Could you check a few things on this model? Use its own coordinates, in mm. Round coordinates to 2 decimals unless told otherwise and drop trailing zeros. Write each loop counter-clockwise with the first axis right and the second up, starting at its lowest first coordinate (ties: lowest second). Pieces come first, ordered by that corner, then holes.
```python
from build123d import *

# Parameters (mm, degrees)
EXTRUDE_START        = 90
SKETCH_1_R           = 1.65
EXTRUDE_262_DEPTH    = 2
EXTRUDE_START_2      = 4
EXTRUDE_1_DEPTH      = 4
D3P2_1_START         = 2
SKETCH_3_R           = 1.6
D3P2_1_DEPTH         = 2
EXTRUDE_1_2_DEPTH    = 4
SKETCH_5_R           = 1.6
D3P2_1_2_DEPTH       = 2
CUT_EXTRUDE_START    = 90
CUT_EXTRUDE_45_DEPTH = 2


with BuildPart() as part:
    # 草图1 → Extrude 262 (new body)
    with BuildSketch(Plane(origin=(0, 0, 0), x_dir=(1, 0, 0), z_dir=(0, 1, 0)).offset(EXTRUDE_START)):
        Polygon((-22.5, -3.5), (-22.5, -12), (-24.25, -15), (-24.25, -53), (-21.25, -56), (-5, -56), (-5, -59), (5, -59), (5, -56), (21.25, -56), (24.25, -53), (24.25, -15), (22.5, -12), (22.5, -3.5), align=None)
        with Locations(Location((0, -56.5, 0), (0, 0, 270))):
            Circle(SKETCH_1_R, mode=Mode.SUBTRACT)
    extrude(amount=EXTRUDE_262_DEPTH)

    # 草图2 → Extrude 1 (add)
    with BuildSketch(Plane.XY.offset(EXTRUDE_START_2)):
        with BuildLine():
            Line((-20.5, 88), (-15.5, 88))
            ThreePointArc((-15.5, 88), (-15.146446609, 88.146446609), (-15, 88.5))
            Line((-15, 88.5), (-15, 89.5))
            ThreePointArc((-15, 89.5), (-15.146446609, 89.853553391), (-15.5, 90))
            Line((-15.5, 90), (-20.5, 90))
            ThreePointArc((-20.5, 90), (-20.853553391, 89.853553391), (-21, 89.5))
            Line((-21, 89.5), (-21, 88.5))
            ThreePointArc((-21, 88.5), (-20.853553391, 88.146446609), (-20.5, 88))
        make_face()
    extrude(amount=EXTRUDE_1_DEPTH)

    # 草图3 → D3p2_-1 (add)
    with BuildSketch(Plane.XY.offset(D3P2_1_START)):
        with Locations(Location((-18, 89, 0), (0, 0, 218.682187453))):
            Circle(SKETCH_3_R)
    extrude(amount=D3P2_1_DEPTH)

    # 草图4 → Extrude 1 2 (add)
    with BuildSketch(Plane.XY.offset(EXTRUDE_START_2)):
        with BuildLine():
            Line((15.5, 88), (20.5, 88))
            ThreePointArc((20.5, 88), (20.853553391, 88.146446609), (21, 88.5))
            Line((21, 88.5), (21, 89.5))
            ThreePointArc((21, 89.5), (20.853553391, 89.853553391), (20.5, 90))
            Line((20.5, 90), (15.5, 90))
            ThreePointArc((15.5, 90), (15.146446609, 89.853553391), (15, 89.5))
            Line((15, 89.5), (15, 88.5))
            ThreePointArc((15, 88.5), (15.146446609, 88.146446609), (15.5, 88))
        make_face()
    extrude(amount=EXTRUDE_1_2_DEPTH)

    # 草图5 → D3p2_1 2 (add)
    with BuildSketch(Plane.XY.offset(D3P2_1_START)):
        with Locations(Location((18, 89, 0), (0, 0, 218.682187453))):
            Circle(SKETCH_5_R)
    extrude(amount=D3P2_1_2_DEPTH)

    # 草图6 → 后盖45度平行通气孔 (cut)
    with BuildSketch(Plane(origin=(0, 0, 0), x_dir=(1, 0, 0), z_dir=(0, 1, 0)).offset(CUT_EXTRUDE_START)):
        with BuildLine():
            Line((-1.767766953, -21.464466094), (3.535533906, -26.767766953))
            ThreePointArc((3.535533906, -26.767766953), (3.535533906, -28.535533906), (1.767766953, -28.535533906))
            Line((1.767766953, -28.535533906), (-3.535533906, -23.232233047))
            ThreePointArc((-3.535533906, -23.232233047), (-3.535533906, -21.464466094), (-1.767766953, -21.464466094))
        make_face()
        with BuildLine():
            Line((-1.767766953, -27.464466094), (3.535533906, -32.767766953))
            ThreePointArc((3.535533906, -32.767766953), (3.535533906, -34.535533906), (1.767766953, -34.535533906))
            Line((1.767766953, -34.535533906), (-3.535533906, -29.232233047))
            ThreePointArc((-3.535533906, -29.232233047), (-3.535533906, -27.464466094), (-1.767766953, -27.464466094))
        make_face()
    extrude(amount=CUT_EXTRUDE_45_DEPTH, mode=Mode.SUBTRACT)


solid = part.part
```
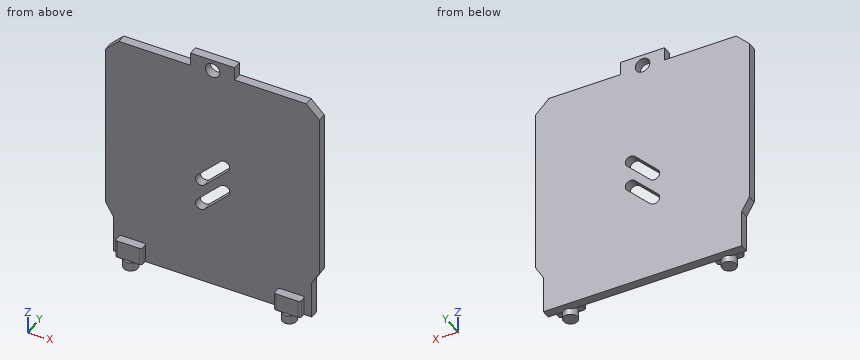
Q1. Imagine slicing it at D-D, the plane z = 19. Write out the boundary of the cut face in (x, y).
Q2. Imagine slicing it at A-A, the plane x = 0. Write out the boundary of the cut face in (y, z).
Q3. I'm going to push flat-ended pins straight in: pin 1 Ø0.6 at (x, y) = (13.5, 90.5) entering from +Z; pin 2 Ø1.6 at (y, z) = (90.5, 57) entering from +X; pin 3 Ø2 at (y, z) = (91, 9) entering from +X. Where does each tip first touch, or does it pass through?
Q4. Imagine slicing it at C-C, the plane x = -18. Write out the boundary of the cut face in (y, z), then the cut area to 3 significant figures.
Q5. Imagine slicing it at B-B, the plane z = 25. Write out the boundary of the cut face in (x, y), then the cut area to 3 significant figures.
Q6. If I drill on L1, parallel to X at y = 91.15, z = 56.5; L2, parallel to X at y = 88.95, z = 6; L3, parallel to Y at x = -4, z = 51, over which ranges is the centre line in solid material (lowest first)?
Results found:
1. outline: (-24.25, 90) - (24.25, 90) - (24.25, 92) - (-24.25, 92) - close
2. outline: (90, 3.5) - (92, 3.5) - (92, 23.23) - (90, 23.23) - close; (90, 26.77) - (92, 26.77) - (92, 29.23) - (90, 29.23) - close; (90, 32.77) - (92, 32.77) - (92, 54.85) - (90, 54.85) - close; (90, 58.15) - (92, 58.15) - (92, 59) - (90, 59) - close
3. pin 1: stops at z = 56
3. pin 2: stops at x = 5
3. pin 3: stops at x = 22.5
4. outline: (87.4, 2) - (90.6, 2) - (90.6, 3.5) - (92, 3.5) - (92, 56) - (90, 56) - (90, 8) - (88, 8) - (88, 4) - (87.4, 4) - close
4. area: 119 mm2
5. outline: (-24.25, 90) - (-1.77, 90) - (-1.77, 92) - (-24.25, 92) - close; (1.77, 90) - (24.25, 90) - (24.25, 92) - (1.77, 92) - close
5. area: 89.9 mm2
6. L1: x = -5 to -1.65, 1.65 to 5
6. L2: x = -21 to -15, 15 to 21
6. L3: y = 90 to 92
